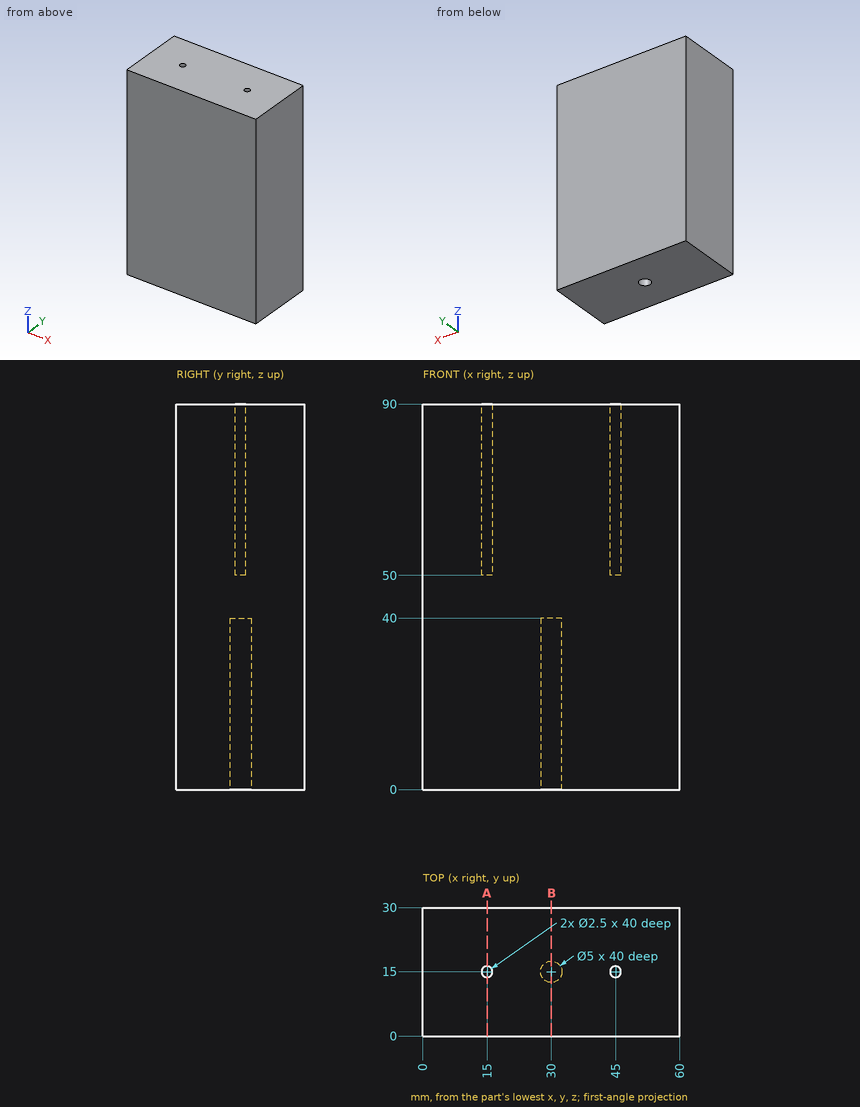
The drawing under review shows one solid part. Ordinate dimensions are in mm from its lowest x, y, z. Coordinates: 2 decimals unless noted, no trailing zeros. Order: outer loops, then holes, each group sorted by start corner. A loop starts at its lowest first (then second) coordinate and runs counter-clockwise, first axis right, second up. Notation, with made-up numbers: (43, 36.5) -> (98, 36.5) arc R12 cw to (98, 40.5) -> close; hole circle Ø10 at (-23.75, 35). An arc over 180 degrees is marked (long way). Answer in a Markdown table with one row per item. Add a question column.
Item 1: We need section A-A on x = 15. Write out the cut boundary in (y, z), plus the area to 3 significant figures.
Item 2: We need section B-B on x = 30. Write out the cut boundary in (y, z), plus the area to 3 significant figures.
Item 3: Clearance check with flat-ended pins moving along their axes: pin 1 (1.2 mm diameter, centred on x = 14.5, y = 15.5, fed in from +Z); pin 2 (2.5 mm diameter, centred on x = 30.5, y = 14, fed in from -Z); pin 3 (0.8 mm diameter, centred on x = 44.5, y = 14.5, fed in from +Z). State where each tip first meets the part, or that it passes through.
Item 4: To check wall thickness, follow probe 1 along Y at (x, z) = (15, 68); probe 2 along Y at (x, z) = (30, 23.5); probe 3 along X at (y, z) = (15.25, 27.5). State the ranges of each line that lie inside material, in increasing order.
Final values:
| question | item | result |
|---|---|---|
| 1 | outline | (0, 0) -> (30, 0) -> (30, 90) -> (16.25, 90) -> (16.25, 50) -> (13.75, 50) -> (13.75, 90) -> (0, 90) -> close |
| 1 | area | 2,600 mm2 |
| 2 | outline | (0, 0) -> (12.5, 0) -> (12.5, 40) -> (17.5, 40) -> (17.5, 0) -> (30, 0) -> (30, 90) -> (0, 90) -> close |
| 2 | area | 2,500 mm2 |
| 3 | pin 1 | stops at z = 90 |
| 3 | pin 2 | stops at z = 40 |
| 3 | pin 3 | stops at z = 50 |
| 4 | probe 1 | y = 0 to 13.75, 16.25 to 30 |
| 4 | probe 2 | y = 0 to 12.5, 17.5 to 30 |
| 4 | probe 3 | x = 0 to 27.51, 32.49 to 60 |
